Input: part model. Units: mm. Frame: model coordinates. Face numbers are marked on the shaded views. Round coordinates to 2 decimals unless told otherwise and drop trailing zeros. Loops run counter-clockwise (first coordinate to the right, second up) from the corner with the lowest first, then second, coordinate; pieces in that order, holes last.
1) Section A-A, the plane x = 9. Return loops of the section in (y, z).
2) Ray query, line 1 along Y through (x, z) = (7.25, 0); line 2 along Z through (x, y) = (6.5, -2.75); line 3 along Y through (x, z) = (10, 1.75). Return the intervals inside material, ascending.
3) Section B-B, the plane x = 2. Return loops of the section in (y, z), and give its area (3 significant figures).
4) First-contact query: pin 1 (2 mm diameter, centred on x = 10.5, y = 4.5, fed in from +Z); pin 2 (3 mm diameter, centred on x = 8, z = -3, fed in from +Y); pin 3 (6 mm diameter, centred on y = -1, z = 4, fed in from -X). Flat tips, straight axial feed; report the tip coordinate or a pass-through.
5) Draft query along Z for the marked faces 1, 2 and 3. Return one class per face: pulls with the +Z half, pulls with the -Z half, needs draft (parallel to the pull), parting line crosses it, or undercut.
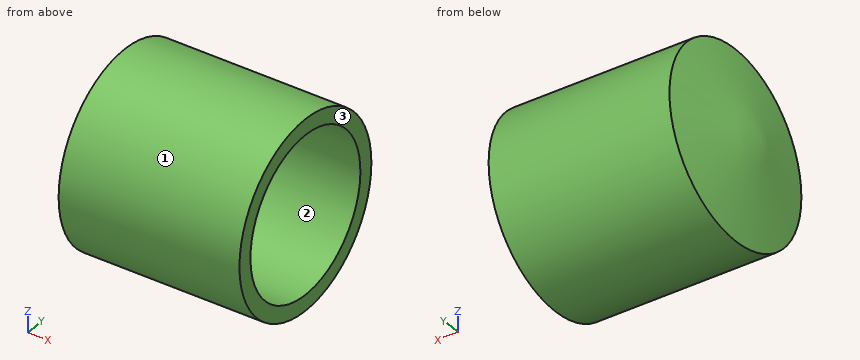
from build123d import *

# Parameters (mm, degrees)
SKETCH_1_R      = 6
EXTRUDE_1_DEPTH = 13
SHELL_1_T       = -1


with BuildPart() as part:
    # 草圖1 → 填料-伸長1 (new body)
    with BuildSketch(Plane(origin=(0, 0, 0), x_dir=(0, 0, -1), z_dir=(1, 0, 0))):
        with Locations(Location((0, 0, 0), (0, 0, 180))):
            Circle(SKETCH_1_R)
    extrude(amount=EXTRUDE_1_DEPTH)

    # 草圖2 → 除料-旋轉2 (revolve, cut)
    with BuildSketch(Plane(origin=(0, 0, 0), x_dir=(1, 0, 0), z_dir=(0, 1, 0)), mode=Mode.PRIVATE) as cut_revolve_2_sk:
        Polygon((0, 0), (1.5, 6), (1.5, 6.496398709), (-0.462606834, 6.496398709), (-0.462606834, 0), align=None)
    revolve(cut_revolve_2_sk.sketch.rotate(Axis((1.002912705, 0, 0), (-1, 0, 0)), 180), axis=Axis((1.002912705, 0, 0), (-1, 0, 0)), mode=Mode.SUBTRACT)

    # 薄殼1
    shell_1_openings = [part.faces().sort_by_distance(p)[0] for p in [
        (13, 0, 0),
    ]]
    offset(amount=SHELL_1_T, openings=shell_1_openings, kind=Kind.INTERSECTION)


solid = part.part
Final values:
1. outline: circle Ø12 at (0, 0); hole circle Ø10 at (0, 0)
2. line 1: y = -6 to -5, 5 to 6
2. line 2: z = -5.33 to -4.18, 4.18 to 5.33
2. line 3: y = -5.74 to -4.68, 4.68 to 5.74
3. outline: circle Ø12 at (0, 0); hole circle Ø7.75 at (0, 0)
3. area: 65.9 mm2
4. pin 1: stops at z = 4.87
4. pin 2: stops at y = 5.81
4. pin 3: stops at x = 0.28
5. face 1: parting line crosses it
5. face 2: undercut
5. face 3: needs draft
